from build123d import *

# Parameters (mm, degrees)
BOSS_EXTRUDE1_DEPTH = 30
SKETCH3_R           = 4.1
CUT_EXTRUDE1_DEPTH  = 81.160460929
SKETCH4_R           = 4.1
CUT_EXTRUDE2_DEPTH  = 72.938334134
FILLET1_R           = 7
SKETCH6_W           = 10
SKETCH6_H           = 50
CUT_EXTRUDE3_DEPTH  = 71.426013762


with BuildPart() as part:
    # Sketch1 → Boss-Extrude1 (new body)
    with BuildSketch(Plane(origin=(0, 0, 0), x_dir=(1, 0, 0), z_dir=(0, 1, 0))):
        Polygon((-22.986013986, 8.601398601), (-22.986013986, -11.398601399), (-5.986013986, -11.398601399), (-5.986013986, -2.307692308), (8.013986014, -2.307692308), (8.013986014, -11.398601399), (25.013986014, -11.398601399), (25.013986014, 8.601398601), (6.013986014, 8.601398601), (6.013986014, 58.601398601), (-3.986013986, 58.601398601), (-3.986013986, 8.601398601), align=None)
    extrude(amount=BOSS_EXTRUDE1_DEPTH)

    # Sketch3 → Cut-Extrude1 (cut, through all)
    with BuildSketch(Plane.XY.offset(11.398601399)):
        with Locations((-14.486013986, 15)):
            Circle(SKETCH3_R)
        with Locations((16.513986014, 15)):
            Circle(SKETCH3_R)
    extrude(amount=-CUT_EXTRUDE1_DEPTH, mode=Mode.SUBTRACT)

    # Sketch4 → Cut-Extrude2 (cut, through all)
    with BuildSketch(Plane(origin=(6.013986014, 0, 0), x_dir=(0, 0, -1), z_dir=(1, 0, 0))):
        with Locations((28.601398601, 15)):
            Circle(SKETCH4_R)
        with Locations((48.601398601, 15)):
            Circle(SKETCH4_R)
    extrude(amount=-CUT_EXTRUDE2_DEPTH, mode=Mode.SUBTRACT)

    # Fillet1
    fillet1_edges = [part.edges().sort_by_distance(p)[0] for p in [
        (-5.986013986, 15, 2.307692308),
        (8.013986014, 15, 2.307692308),
    ]]
    fillet(fillet1_edges, radius=FILLET1_R - 0.0001)  # a hair under: the kernel refuses the full size

    # Sketch6 → Cut-Extrude3 (cut, through all)
    with BuildSketch(Plane(origin=(0, 30, 0), x_dir=(1, 0, 0), z_dir=(0, 1, 0))):
        with Locations((1.013986014, 33.601398601)):
            Rectangle(SKETCH6_W, SKETCH6_H)
    extrude(amount=-CUT_EXTRUDE3_DEPTH, mode=Mode.SUBTRACT)


solid = part.part
Work out the finished part from the listing and answer in its coordinate system (mm). A direction names the side the tool comes from. Round coordinates to 2 decimals unless told otherwise and drop trailing zeros. Write each loop counter-clockwise with the first axis right and the second up, starting at its lowest first coordinate (ties: lowest second). Pieces come first, ordered by that corner, then holes.
1) A tool of negligible diameter and unlimited length cuts with its end or side. For faces 5 (the flat face through (-5.986, 15, 10)), 6 (the flat face through (-18, 18, 11.399)), from which of +Z, -Z, +X, -X, +Y, -Y can it reach the whole face along a straight path? Write none if from no direction.
2) A cutting plane is placed at A-A (z = 7). Give the vertices of the cut face in (x, y).
3) Straight lines are drawn through the part: line 1 (Y direction, x = 16.5, z = -6.5); line 2 (X direction, y = 11.5, z = 8.75); line 3 (X direction, y = 3.5, z = 9.5). For each, find the intervals that lie inside material, in ascending order.
4) A cutting plane is placed at B-B (y = 15). Give the number of separate pieces and of enclosed holes in the cut face, plus the area to 3 significant figures.
5) A cutting plane is placed at D-D (z = -1.25). Give the vertices of the cut face in (x, y), plus the area to 3 significant figures.
6) The mould has two halves that part along X. Classify faces 1 (the flat face through (1, 0, 1)), 2 (the flat face through (8.014, 15, 10)), 3 (the flat face through (-22.986, 15, 1)), 4 (the cylindrical face through (5.909, 15.21, 4.304)): pulls with the +X half, pulls with the -X half, needs draft (parallel to the pull), parting line crosses it, or undercut.
Completed:
1. face 5: +Z, +Y, -Y
1. face 6: +Z, +X, -X, +Y, -Y
2. outline: (-22.99, 0) - (-5.59, 0) - (-5.59, 30) - (-22.99, 30) - close; (7.62, 0) - (25.01, 0) - (25.01, 30) - (7.62, 30) - close; hole circle Ø8.2 at (-14.49, 15); hole circle Ø8.2 at (16.51, 15)
3. line 1: y = 0 to 10.9, 19.1 to 30
3. line 2: x = -22.99 to -16.62, -12.35 to -5.96, 7.99 to 14.38, 18.65 to 25.01
3. line 3: x = -22.99 to -5.99, 8.01 to 25.01
4. separate pieces: 3
4. enclosed holes: 0
4. area: 526 mm2
5. outline: (-22.99, 0) - (25.01, 0) - (25.01, 30) - (-22.99, 30) - close; hole circle Ø8.2 at (-14.49, 15); hole circle Ø8.2 at (16.51, 15)
5. area: 1,330 mm2
6. face 1: needs draft
6. face 2: undercut
6. face 3: pulls with the -X half
6. face 4: undercut
